Geometry check sheet. Reference: the model listing, model coordinates, mm. A direction names the side the tool comes from. Round coordinates to 2 decimals unless told otherwise and drop trailing zeros. Loops run counter-clockwise (first coordinate to the right, second up) from the corner with the lowest first, then second, coordinate; pieces in that order, holes last. Notation, with made-up numbers: M 54.25,-10 L 61.25,-10 A16 cw 61.25,19 Z; hole C -28,-5 d3. An arc over 180 degrees is marked long. Use one line per item in the form item = value. Start each with the question number.
1. Cross-section at A-A (y = 0). Record the boundary of the cut face in (x, z).
2. Material ranges on line 1 (Y direction, x = 0, z = 13); line 2 (Z direction, x = -1.5, y = -0.75); line 3 (X direction, y = -1, z = -21), recorded low to high.
3. Set-up check for faces 4 (the flat face through (3.4, -1.7, -30)), 5 (the cylindrical face through (3.233, 1.341, -15.703)), 6 (the cylindrical face through (3.233, -1.341, 15.703)): record each of +Z, -Z, +X, -X, +Y, -Y from which the full face is reachable in a straight line by a thin tool's end or side.
4. Cross-section at C-C (z = -5.5). Record the boundary of the cut face in (x, y), then the cut area to 3 significant figures.
5. Go/stop test with flat-tipped pins: pin 1 (2 mm diameter, centred on x = 1.5, y = 0.5, fed in from +Z); pin 2 (3 mm diameter, centred on y = 6, z = 20, fed in from +X); pin 3 (2 mm diameter, centred on x = -6, z = -10, fed in from +Y). Record where each tip stops, or that it passes through.
6. Draft check along Y on faces 1 (the cylindrical face through (-2.17, -9.76, 0.39)), 2 (the flat face through (3.4, -1.7, 30)), 3 (the flat face through (0, 0, -1)). Enter one of: pulls with the +Y half, pulls with the -Y half, needs draft (parallel to the pull), parting line crosses it, or undercut.
```python
from build123d import *

# Parameters (mm, degrees)
F0_R     = 10
F1_DEPTH = 30
F2_R     = 3.5
F4_DEPTH = 29
F3_R     = 3.5
F5_DEPTH = 29
F6_SIZE  = 2


with BuildPart() as f1:
    # F0 (on Top) → F1 (new body, symmetric)
    with BuildSketch(Plane.XY):
        Circle(F0_R)
    extrude(amount=F1_DEPTH, both=True)

    # F2 (on face) → F4 (cut)
    with BuildSketch(Plane(origin=(0, 0, -30), x_dir=(1, 0, 0), z_dir=(0, 0, -1))):
        Circle(F2_R)
    extrude(amount=-F4_DEPTH, mode=Mode.SUBTRACT)

    # F3 (on face) → F5 (cut)
    with BuildSketch(Plane.XY.offset(30)):
        Circle(F3_R)
    extrude(amount=-F5_DEPTH, mode=Mode.SUBTRACT)

    # F6
    f6_edges = [f1.edges().sort_by_distance(p)[0] for p in [
        (-10, 0, 30),
        (-10, 0, -30),
    ]]
    chamfer(f6_edges, length=F6_SIZE)


solid = f1.part
```
Reported:
q1.outline = M -10,-28 L -8,-30 L -3.5,-30 L -3.5,-1 L 3.5,-1 L 3.5,-30 L 8,-30 L 10,-28 L 10,28 L 8,30 L 3.5,30 L 3.5,1 L -3.5,1 L -3.5,30 L -8,30 L -10,28 Z
q2.line_1 = -10 to -3.5, 3.5 to 10
q2.line_2 = -1 to 1
q2.line_3 = -9.95 to -3.35, 3.35 to 9.95
q3.face_4 = -Z, +X, -X, +Y, -Y
q3.face_5 = -Z
q3.face_6 = +Z
q4.outline = C 0,0 d20; hole C 0,0 d7
q4.area = 276 mm²
q5.pin_1 = 1
q5.pin_2 = 8.93
q5.pin_3 = 8.66
q6.face_1 = parting line crosses it
q6.face_2 = needs draft
q6.face_3 = undercut
